Read the model definition and answer for the solid it produces. Units are mm, in the model's axes. Face numbers are marked on the shaded views. A direction names the side the tool comes from. Coordinates: 2 decimals unless noted, no trailing zeros. Write each loop counter-clockwise with the first axis right and the second up, starting at its lowest first coordinate (ties: lowest second). Pieces come first, ordered by that corner, then holes. Notation, with made-up numbers: (-10, 75) -> (29, 75) arc R21 ccw to (29, 82) -> close; hole circle Ø10 at (-37, 5). An arc over 180 degrees is marked (long way). Answer in a Markdown table with one row per item. Add a question column.
Item 1: For a pull along Y with two mould halves and no side action, classify the marked faces 1, 2, 3 and 4 as +Y half, -Y half, draft (parallel to the pull), parting line (faces both ways), or undercut.
Item 2: Section C-C on z = 23.5 is taken. Write down the section's boundary in (x, y), then the cut area to 3 significant figures.
Item 3: Straight lines are drawn through the part: line 1 (Y direction, x = -1, z = 5.5); line 2 (X direction, y = -1, z = 5.25); line 3 (Z direction, x = 12.5, y = -7.5). For each, find the intervals that lie inside material, in ascending order. Write a range as from..to.
Item 4: Which of the six approach directions +Z, -Z, +X, -X, +Y, -Y give full straight-line access (tool end or side, diameter ignored) to the marked faces 5, 6, 7, 8 and 9?
Item 5: Section D-D on y = -9.5 is taken. Write down the section's boundary in (x, z).
Item 6: Section B-B on x = 6.5 is taken. Write down the section's boundary in (y, z), then the cut area to 3 significant figures.
Item 7: Given pin 1 Ø1.9 at (y, z) = (14.5, 7.5) entering from +X; pin 2 Ø3 at (x, y) = (0, 19) entering from -Z; pin 3 Ø4 at (x, z) = (-4, 10) entering from +Y, each flat-ended and moving along its own axis, determine where each tip first touches the part or whether it passes through.
Item 8: Section A-A on z = 10.25 is taken. Write down the section's boundary in (x, y), then the cut area to 3 significant figures.
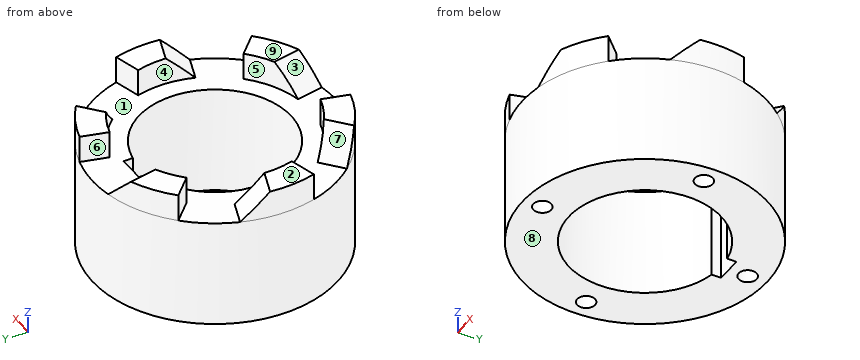
```python
from build123d import *

# Parameters (mm, degrees)
SKETCH1_R                    = 22.5
BOSS_EXTRUDE1_DEPTH          = 20
BOSS_EXTRUDE2_DEPTH          = 5
CHAMFER2_SIZE                = 5
CIRPATTERN1_COUNT            = 6
CHAMFER2_OF_CIRPATTERN1_SIZE = 5
CIRPATTERN2_COUNT            = 4


with BuildPart() as part:
    # Sketch1 → Boss-Extrude1 (new body)
    with BuildSketch(Plane.XY):
        Circle(SKETCH1_R)
        with BuildLine():
            Line((2.5, 15.5), (-2.5, 15.5))
            Line((-2.5, 15.5), (-2.5, 13.774977314))
            ThreePointArc((-2.5, 13.774977314), (0, -14), (2.5, 13.774977314))
            Line((2.5, 13.774977314), (2.5, 15.5))
        make_face(mode=Mode.SUBTRACT)
    extrude(amount=BOSS_EXTRUDE1_DEPTH)

    # Sketch2 → Boss-Extrude2 (add)
    with BuildSketch(Plane.XY.offset(20)):
        with BuildLine():
            Line((-3.189121696, 17.206960882), (-4.100299324, 22.12323542))
            ThreePointArc((-4.100299324, 22.12323542), (-10.476326707, 19.912221843), (-15.909902577, 15.909902577))
            Line((-15.909902577, 15.909902577), (-12.374368671, 12.374368671))
            ThreePointArc((-12.374368671, 12.374368671), (-8.148254106, 15.487283656), (-3.189121696, 17.206960882))
        make_face()
    boss_extrude2 = extrude(amount=BOSS_EXTRUDE2_DEPTH)

    # Chamfer2
    chamfer2_edges = [part.edges().sort_by_distance(p)[0] for p in [
        (-3.64471051, 19.665098151, 25),
    ]]
    chamfer(chamfer2_edges, length=CHAMFER2_SIZE - 0.0001)  # a hair under: the kernel refuses the full size

    # CirPattern1: Boss-Extrude2 ×6 about axis
    cirpattern1_axis = Axis((0, 0, 0), (0, 0, 1))
    for i in range(1, CIRPATTERN1_COUNT):
        add(boss_extrude2.rotate(cirpattern1_axis, i * 360 / CIRPATTERN1_COUNT))

    # Chamfer2 of CirPattern1
    chamfer2_of_cirpattern1_edges = [part.edges().sort_by_distance(p)[0] for p in [
        (-18.852829822, 6.676137185, 25),
        (-15.208119312, -12.988960967, 25),
        (3.64471051, -19.665098151, 25),
        (18.852829822, -6.676137185, 25),
        (15.208119312, 12.988960967, 25),
    ]]
    chamfer(chamfer2_of_cirpattern1_edges, length=CHAMFER2_OF_CIRPATTERN1_SIZE - 0.0001)  # a hair under: the kernel refuses the full size

    # Sketch4 → M4 Tapped Hole1 (revolve, cut)
    with BuildSketch(Plane(origin=(0, 19, 0), x_dir=(0, 1, 0), z_dir=(1, 0, 0))):
        Polygon((0, 0), (0, 12.491420021), (1.65, 11.5), (1.65, 0), align=None)
    m4_tapped_hole1 = revolve(axis=Axis((0, 19, -6.35), (0, 0, 1)), mode=Mode.SUBTRACT)

    # CirPattern2: M4 Tapped Hole1 ×4 about axis
    cirpattern2_axis = Axis((0, 0, 0), (0, 0, 1))
    for i in range(1, CIRPATTERN2_COUNT):
        add(m4_tapped_hole1.rotate(cirpattern2_axis, i * 360 / CIRPATTERN2_COUNT), mode=Mode.SUBTRACT)


solid = part.part
```
Results below:
| question | item | result |
|---|---|---|
| 1 | face 1 | undercut |
| 1 | face 2 | draft |
| 1 | face 3 | -Y half |
| 1 | face 4 | undercut |
| 2 | outline | (-22.12, 4.12) arc R22.5 ccw to (-21.73, -5.82) -> (-16.9, -4.53) arc R17.5 cw to (-17.33, 2.42) -> close; (-15.91, 15.91) -> (-12.37, 12.37) arc R17.5 cw to (-6.57, 16.22) -> (-7.49, 21.22) arc R22.5 ccw to start; (-14.63, -17.1) arc R22.5 ccw to (-5.82, -21.73) -> (-4.53, -16.9) arc R17.5 cw to (-10.77, -13.8) -> close; (4.53, 16.9) arc R17.5 cw to (10.77, 13.8) -> (14.63, 17.1) arc R22.5 ccw to (5.82, 21.73) -> close; (6.57, -16.22) -> (7.49, -21.22) arc R22.5 ccw to (15.91, -15.91) -> (12.37, -12.37) arc R17.5 cw to start; (16.9, 4.53) arc R17.5 cw to (17.33, -2.42) -> (22.12, -4.12) arc R22.5 ccw to (21.73, 5.82) -> close |
| 2 | area | 256 mm2 |
| 3 | line 1 | y = -22.48..-20.31, -17.69..-13.96, 15.5..17.69, 20.31..22.48 |
| 3 | line 2 | x = -22.48..-20.31, -17.69..-13.96, 13.96..17.69, 20.31..22.48 |
| 3 | line 3 | z = 0..20 |
| 4 | face 5 | +Z |
| 4 | face 6 | +Z, +Y |
| 4 | face 7 | +Z, -X |
| 4 | face 8 | -Z, +X, -X, +Y, -Y |
| 4 | face 9 | +Z, +X, -X, +Y, -Y |
| 5 | outline | (-20.4, 0) -> (-10.28, 0) -> (-10.28, 20) -> (-20.4, 20) -> close; (10.28, 0) -> (20.4, 0) -> (20.4, 20) -> (10.28, 20) -> close |
| 6 | outline | (-21.54, 0) -> (-12.4, 0) -> (-12.4, 20) -> (-16.25, 20) -> (-16.25, 23.43) -> (-21.54, 22.47) -> close; (12.4, 0) -> (21.54, 0) -> (21.54, 25) -> (16.25, 25) -> (16.25, 20) -> (12.4, 20) -> close |
| 6 | area | 408 mm2 |
| 7 | pin 1 | stops at x = 17.96 |
| 7 | pin 2 | stops at z = 11.59 |
| 7 | pin 3 | stops at y = 22.41 |
| 8 | outline | circle Ø45 at (0, 0); hole circle Ø3.3 at (-19, 0); hole (-2.5, 13.77) arc R14 ccw (long way) to (2.5, 13.77) -> (2.5, 15.5) -> (-2.5, 15.5) -> close; hole circle Ø3.3 at (0, -19); hole circle Ø3.3 at (0, 19); hole circle Ø3.3 at (19, 0) |
| 8 | area | 933 mm2 |
